Geometry check sheet. Reference: the model listing, model coordinates, mm. Face numbers are marked on the shaded views. A direction names the side the tool comes from. Round coordinates to 2 decimals unless told otherwise and drop trailing zeros. Write each loop counter-clockwise with the first axis right and the second up, starting at its lowest first coordinate (ties: lowest second). Pieces come first, ordered by that corner, then holes. Notation, with made-up numbers: (-12, 5.25) - (1, 5.25) arc R25 cw to (1, 25.25) - close; hole circle Ø8 at (79.25, -13.75). An arc over 180 degrees is marked (long way). Return JSON: item names as keys, results as strings.
```python
from build123d import *

# Parameters (mm, degrees)
SKETCH1_W                    = 12
SKETCH1_H                    = 10.5
BASE_DEPTH                   = 8.25
CONTACT_OPENING_DEPTH        = 9
CONTACT_OPENING_LEAD_IN_SIZE = 0.5
SKETCH3_W                    = 5.6
SKETCH3_H                    = 3.18
CONTACT_AREA_DEPTH           = 8.5
CONTACT_AREA_LEAD_IN_SIZE    = 0.5
HOLDING_TINES_DEPTH          = 1.75
CONTACT_DEPTH                = 0.375
CONTACT_PATTERN_COUNT        = 2
CONTACT_PATTERN_PITCH        = 2.5
BOSS_EXTRUDE1_DEPTH          = 6.75
CHAMFER1_SIZE                = 6
SKETCH17_R                   = 1.5
CUT_EXTRUDE1_DEPTH           = 27.5
CUT_EXTRUDE2_DEPTH           = 27.5
FILLET1_R                    = 2
SKETCH20_R                   = 4.5
BOSS_EXTRUDE2_DEPTH          = 3
SKETCH21_R                   = 2.5
BOSS_EXTRUDE3_DEPTH          = 10


with BuildPart() as part:
    # Sketch1 → Base (new body, symmetric)
    with BuildSketch(Plane.XY):
        Rectangle(SKETCH1_W, SKETCH1_H)
    extrude(amount=BASE_DEPTH, both=True)

    # Sketch2 → Contact Opening (cut)
    with BuildSketch(Plane.XY.offset(8.25)):
        with BuildLine():
            Line((-2.975, 4.33), (-4.225, 3.08))
            Line((-4.225, 3.08), (-4.225, -2.95))
            ThreePointArc((-4.225, -2.95), (-4.078553391, -3.303553391), (-3.725, -3.45))
            Line((-3.725, -3.45), (3.725, -3.45))
            ThreePointArc((3.725, -3.45), (4.078553391, -3.303553391), (4.225, -2.95))
            Line((4.225, -2.95), (4.225, 3.08))
            Line((4.225, 3.08), (2.975, 4.33))
            Line((2.975, 4.33), (-2.975, 4.33))
        make_face()
    extrude(amount=-CONTACT_OPENING_DEPTH, mode=Mode.SUBTRACT)

    # Contact Opening Lead-in
    contact_opening_lead_in_edges = [part.edges().sort_by_distance(p)[0] for p in [
        (0, 4.33, 8.25),
        (-3.6, 3.705, 8.25),
        (-4.225, 0.065, 8.25),
        (-4.078553391, -3.303553391, 8.25),
        (0, -3.45, 8.25),
        (4.078553391, -3.303553391, 8.25),
        (4.225, 0.065, 8.25),
        (3.6, 3.705, 8.25),
    ]]
    chamfer(contact_opening_lead_in_edges, length=CONTACT_OPENING_LEAD_IN_SIZE)

    # Sketch3 → Contact Area (add)
    with BuildSketch(Plane.XY.offset(-0.75)):
        with Locations((0, 0.44)):
            Rectangle(SKETCH3_W, SKETCH3_H)
    extrude(amount=CONTACT_AREA_DEPTH)

    # Contact Area Lead-in
    contact_area_lead_in_edges = [part.edges().sort_by_distance(p)[0] for p in [
        (-2.8, 0.44, 7.75),
        (0, -1.15, 7.75),
        (2.8, 0.44, 7.75),
        (0, 2.03, 7.75),
    ]]
    chamfer(contact_area_lead_in_edges, length=CONTACT_AREA_LEAD_IN_SIZE)

    # Sketch7 → Holding Tines (add, symmetric)
    with BuildSketch(Plane(origin=(0, 0, 0), x_dir=(1, 0, 0), z_dir=(0, 1, 0))):
        with BuildLine():
            Line((-4.225, -7.75), (-3.215243234, -5.051316752))
            ThreePointArc((-3.215243234, -5.051316752), (-3.027350135, -3.881276433), (-3.307189725, -2.729760924))
            Line((-3.307189725, -2.729760924), (-3.695, -1.9))
            Line((-3.695, -1.9), (-3.853538933, -1.974097279))
            Line((-3.853538933, -1.974097279), (-3.465728658, -2.803858203))
            ThreePointArc((-3.465728658, -2.803858203), (-3.202213044, -3.888201975), (-3.379145712, -4.989989942))
            Line((-3.379145712, -4.989989942), (-4.388902478, -7.688673189))
            Line((-4.388902478, -7.688673189), (-4.225, -7.75))
        make_face()
        with BuildLine():
            Line((4.225, -7.75), (4.388902478, -7.688673189))
            Line((4.388902478, -7.688673189), (3.379145712, -4.989989942))
            ThreePointArc((3.379145712, -4.989989942), (3.202213044, -3.888201975), (3.465728658, -2.803858203))
            Line((3.465728658, -2.803858203), (3.853538933, -1.974097279))
            Line((3.853538933, -1.974097279), (3.695, -1.9))
            Line((3.695, -1.9), (3.307189725, -2.729760924))
            ThreePointArc((3.307189725, -2.729760924), (3.027350135, -3.881276433), (3.215243234, -5.051316752))
            Line((3.215243234, -5.051316752), (4.225, -7.75))
        make_face()
    extrude(amount=HOLDING_TINES_DEPTH, both=True)

    # Sketch8 → Contact (add, symmetric)
    with BuildSketch(Plane(origin=(-1.25, 0, 0), x_dir=(0, 0, -1), z_dir=(1, 0, 0))):
        with BuildLine():
            Line((0.75, 2.03), (-2.695251124, 2.678262825))
            ThreePointArc((-2.695251124, 2.678262825), (-3.57053143, 2.712827451), (-4.418484282, 2.493086043))
            Line((-4.418484282, 2.493086043), (-5.75, 1.93))
            Line((-5.75, 1.93), (-5.681838417, 1.768819981))
            Line((-5.681838417, 1.768819981), (-4.350322699, 2.331906024))
            ThreePointArc((-4.350322699, 2.331906024), (-3.551833763, 2.538829183), (-2.727611475, 2.506280827))
            Line((-2.727611475, 2.506280827), (0.717639649, 1.858018002))
            Line((0.717639649, 1.858018002), (0.75, 2.03))
        make_face()
        with BuildLine():
            Line((-5.681838417, -0.888819981), (-5.75, -1.05))
            Line((-5.75, -1.05), (-4.418484282, -1.613086043))
            ThreePointArc((-4.418484282, -1.613086043), (-3.57053143, -1.832827451), (-2.695251124, -1.798262825))
            Line((-2.695251124, -1.798262825), (0.75, -1.15))
            Line((0.75, -1.15), (0.717639649, -0.978018002))
            Line((0.717639649, -0.978018002), (-2.727611475, -1.626280827))
            ThreePointArc((-2.727611475, -1.626280827), (-3.551833763, -1.658829183), (-4.350322699, -1.451906024))
            Line((-4.350322699, -1.451906024), (-5.681838417, -0.888819981))
        make_face()
    contact = extrude(amount=CONTACT_DEPTH, both=True)

    # Contact Pattern: Contact ×2
    with Locations(*[(i * CONTACT_PATTERN_PITCH, 0, 0) for i in range(1, CONTACT_PATTERN_COUNT)]):
        add(contact)


with BuildPart() as body_2:
    # Sketch16 → Boss-Extrude1 (new body, symmetric)
    with BuildSketch(Plane(origin=(0, 0, 0), x_dir=(1, 0, 0), z_dir=(0, 1, 0))):
        Polygon((-8.75, 1.5), (0, 1.5), (0, 18.75), (-12, 18.75), (-12, -0.75), (-19, -0.75), (-19, -7.75), (-8.75, -7.75), align=None)
    extrude(amount=BOSS_EXTRUDE1_DEPTH, both=True)

    # Chamfer1
    chamfer1_edges = [body_2.edges().sort_by_distance(p)[0] for p in [
        (-12, 0, -18.75),
    ]]
    chamfer(chamfer1_edges, length=CHAMFER1_SIZE)

    # Sketch17 → Cut-Extrude1 (cut, through all)
    with BuildSketch(Plane.XY.offset(7.75)):
        with Locations((-15, 0)):
            Circle(SKETCH17_R)
    extrude(amount=-CUT_EXTRUDE1_DEPTH, mode=Mode.SUBTRACT)

    # Sketch18 → Cut-Extrude2 (cut, through all)
    with BuildSketch(Plane.XY.offset(7.75)):
        with BuildLine():
            ThreePointArc((-19, 0), (-17.828427125, 2.828427125), (-15, 4))
            Line((-15, 4), (-12, 4))
            Line((-12, 4), (-12, 6.75))
            Line((-12, 6.75), (-19, 6.75))
            Line((-19, 6.75), (-19, 0))
        make_face()
        with BuildLine():
            ThreePointArc((-15, -4), (-17.828427125, -2.828427125), (-19, 0))
            Line((-19, 0), (-19, -6.75))
            Line((-19, -6.75), (-12, -6.75))
            Line((-12, -6.75), (-12, -4))
            Line((-12, -4), (-15, -4))
        make_face()
    extrude(amount=-CUT_EXTRUDE2_DEPTH, mode=Mode.SUBTRACT)

    # Fillet1
    fillet1_edges = [body_2.edges().sort_by_distance(p)[0] for p in [
        (-3, 6.75, -18.75),
        (-12, -6.75, -2.5),
        (-12, 6.75, -2.5),
        (-12, 0, -12.75),
        (-9, -6.75, -15.75),
        (-6, 0, -18.75),
        (-9, 6.75, -15.75),
        (-3, -6.75, -18.75),
    ]]
    fillet(fillet1_edges, radius=FILLET1_R)

    # Mirror1: body 2 across plane


with BuildPart() as body_2_1:
    add(body_2.part)
    add(body_2.part.mirror(Plane(origin=(0, 6.75, -18.75), x_dir=(0, 0, 1), z_dir=(-1, 0, 0))))

    # Sketch20 → Boss-Extrude2 (add)
    with BuildSketch(Plane(origin=(0, 0, -18.75), x_dir=(-1, 0, 0), z_dir=(0, 0, -1))):
        Circle(SKETCH20_R)
    extrude(amount=BOSS_EXTRUDE2_DEPTH)

    # Sketch21 → Boss-Extrude3 (add)
    with BuildSketch(Plane(origin=(0, 0, -21.75), x_dir=(-1, 0, 0), z_dir=(0, 0, -1))):
        Circle(SKETCH21_R)
    extrude(amount=BOSS_EXTRUDE3_DEPTH)


with BuildPart() as part_1:
    add(part.part)

    # Combine1: union body 2
    add(body_2_1.part)


solid = part_1.part
```
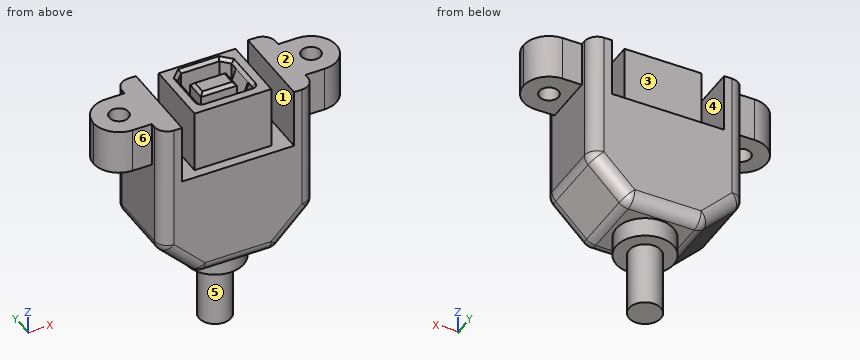
(1) Access from +Z, -Z, +X, -X, +Y, -Y to the whole of each face (thin tool, end or side, straight path). Record for the marked faces 1, 2 and 3.
Response values:
{"face 1": "+Z, +Y, -Y", "face 2": "+Z, +X, +Y, -Y", "face 3": "+Z, +Y"}
(2) Material ranges on line 1 along Y through (x, z) = (15, 3); line 2 along Z through (x, y) = (0.5, -1.5); line 3 along Z through (x, y) = (-14, -3), recorded low to high. Write a range as [from, to].
Response values:
{"line 1": "y = [-4, -1.5], [1.5, 4]", "line 2": "z = [-31.75, -0.75]", "line 3": "z = [0.75, 7.75]"}
(3) Section check B-B, the plane x = 16. Enter the section's corners in (y, z).
Response values:
{"outline": "(-3.87, 0.75) - (-1.12, 0.75) - (-1.12, 7.75) - (-3.87, 7.75) - close; (1.12, 0.75) - (3.87, 0.75) - (3.87, 7.75) - (1.12, 7.75) - close"}
(4) Section check A-A, the plane z = -8. Enter the section's corners in (x, y).
Response values:
{"outline": "(-12, -4.75) arc R2 ccw to (-10, -6.75) - (10, -6.75) arc R2 ccw to (12, -4.75) - (12, 4.75) arc R2 ccw to (10, 6.75) - (-10, 6.75) arc R2 ccw to (-12, 4.75) - close"}
(5) Gauge pin test, flat ends, axial feed: pin 1 (5 mm diameter, centred on y = -5, z = -18, fed in from -X); pin 2 (1.5 mm diameter, centred on y = 3, z = -13, fed in from +X); pin 3 (1.8 mm diameter, centred on x = 15, y = 0, fed in from +Z); pin 4 (1.5 mm diameter, centred on x = 12.5, z = -5, fed in from -Y). Record the tip position at first contact, or that the pin passes through.
Response values:
{"pin 1": "stops at x = -9.24", "pin 2": "stops at x = 11.97", "pin 3": "passes through", "pin 4": "stops at y = -5.72"}
(6) Release check for a two-part mould opening along X. For the marked faces 4, 5 and 6 record: pulls with the +X half, pulls with the -X half, needs draft (parallel to the pull), parting line crosses it, or undercut.
Response values:
{"face 4": "undercut", "face 5": "parting line crosses it", "face 6": "needs draft"}
(7) Section check C-C, the plane y = 5.75. Enter the section's corners in (x, z), plus the area to 3 significant figures.
Response values:
{"outline": "(-11.73, -11.92) arc R1.73 ccw to (-11.22, -13.15) - (-6.4, -17.97) arc R1.73 ccw to (-5.17, -18.48) - (5.17, -18.48) arc R1.73 ccw to (6.4, -17.97) - (11.22, -13.15) arc R1.73 ccw to (11.73, -11.92) - (11.73, 7.75) - (8.75, 7.75) - (8.75, -1.5) - (-8.75, -1.5) - (-8.75, 7.75) - (-11.73, 7.75) - close", "area": "419 mm^2"}
(8) Section check D-D, the plane x = -13. Enter the section's corners in (y, z).
Response values:
{"outline": "(-4, 0.75) - (4, 0.75) - (4, 7.75) - (-4, 7.75) - close"}
